Design review of the part built by this model. Coordinates are the model's own, in mm. A direction names the side the tool comes from. Coordinates: 2 decimals unless noted, no trailing zeros. Order: outer loops, then holes, each group sorted by start corner. A loop starts at its lowest first (then second) coordinate and runs counter-clockwise, first axis right, second up. Notation, with made-up numbers: (51, 33) - (81, 33) arc R19 ccw to (81, 47) - close; hole circle Ø6 at (14.5, 21). An arc over 180 degrees is marked (long way). Write each question's results on one line, items separated by ' | '. Start each with the question number.
```python
from build123d import *

# Parameters (mm, degrees)
F0_W        = 100
F0_H        = 260
F1_DEPTH    = 30
F3_R        = 5
F2_R        = 45
F4_DEPTH    = 20
F5_T        = 5
F5_T4_ANGLE = 180.000000001
F5_T6_ANGLE = 180.000000001


# Not quite as in the source:
# - a shell that OpenCascade refuses in one call is made with other operations: the cavity is built on its own and cut out


with BuildPart() as f1:
    # F0 (on Front) → F1 (new body)
    with BuildSketch(Plane.XZ):
        with Locations((-0.186801888, -30)):
            Rectangle(F0_W, F0_H)
    extrude(amount=-F1_DEPTH)

    # F3
    f3_edges = [f1.edges().sort_by_distance(p)[0] for p in [
        (49.813198, 0, -30),
        (-50.186802, 0, -30),
        (-0.186802, 30, 100),
    ]]
    fillet(f3_edges, radius=F3_R)

    # F2 (on Front) → F4 (join)
    with BuildSketch(Plane.XZ):
        with Locations((-0.186801888, 50)):
            Circle(F2_R)
    extrude(amount=F4_DEPTH)

    # F5: shell of thickness 5, made by hand


with BuildPart() as f5_core1:
    # F5_t2: copy of F1
    add(f1.part)

    # the walls: a layer under each face that stays
    f5_faces = [f5_core1.faces().sort_by_distance(p)[0] for p in [
        (-0.186801888, 12.5, 100),
        (49.813198112, 17.5, -30),
        (-30.186801888, 0, 91.6666666667),
        (-50.186801888, 17.5, -30),
        (-0.186801888, 30, -32.5),
        (-0.186801888, 0, -55),
        (-45.186801888, -10, 50),
        (-0.186801888, -20, 50),
    ]]
    thicken(f5_faces, amount=-F5_T, mode=Mode.SUBTRACT)

    # F5_s3 → F5_t4 (revolve, cut)
    with BuildSketch(Plane.XY.offset(50)):
        Polygon((44.863198112, -0.05), (44.813198112, 5), (39.813198112, 5), (39.813198112, 0), align=None)
    revolve(axis=Axis((-0.186801888, 0, 50), (0, -1, 0)), revolution_arc=F5_T4_ANGLE, mode=Mode.SUBTRACT)

    # F5_s5 → F5_t6 (revolve, cut)
    with BuildSketch(Plane.XY.offset(50)):
        Polygon((-45.236801888, -0.05), (-45.186801888, 5), (-40.186801888, 5), (-40.186801888, 0), align=None)
    revolve(axis=Axis((-0.186801888, 0, 50), (0, -1, 0)), revolution_arc=F5_T6_ANGLE, mode=Mode.SUBTRACT)


with BuildPart() as f1_1:
    add(f1.part)

    # what is left inside the walls is the cavity
    f5_cavity = [f5_core1.part.solids().sort_by_distance(p)[0] for p in [
        (-0.186802, 24.95, -75),
    ]]
    add(f5_cavity, mode=Mode.SUBTRACT)


solid = f1_1.part
```
(1) Clearance check with flat-ended pins moving along their axes: pin 1 (10 mm diameter, centred on x = 8.5, y = 19.5, fed in from -Z); pin 2 (5 mm diameter, centred on x = 24, y = -12, fed in from +Z); pin 3 (3 mm diameter, centred on x = -10.5, z = -130, fed in from -Y). State where each tip first meets the part, or that it passes through.
(2) Take a section at D-D (x = 9). State the section outline as (y, z) points, plus the area to 3 significant figures.
(3) Take a section at B-B (y = 20). State the section outline as (x, z) points.
(4) Take a section at C-C (x = 24). State the section outline as (y, z) points, plus the area to 3 significant figures.
(5) Mouldability with a two-part tool opening along X and no side actions: class faces 6 (the face through (-1, 15, 95)), 7 (the face through (48.387, 1.504, -28.18)), 8 (the face through (-48.76, 1.5, -28.18)), 9 (the face through (-1, 12, 100)) as +X half, -X half, draft (parallel to the pull), parting line (faces both ways), or undercut.
(6) Take a section at A-A (z = -25.5). State the section outline as (x, y) points, plus the area to 3 significant figures.
(7) Tool access review of faces 1 (the face through (-9.94, -9.86, 6.07)), 2 (the face through (-0.4, 0, 95.5)), 3 (the face through (-1, 30, -31)), 4 (the face through (-1, -15, 51)), 5 (the face through (-1, 5, -59)): name each direction out of +Z, -Z, +X, -X, +Y, -Y from which nothing blocks a thin tool from reaching the whole face with its end or side.
(8) To check wall thickness, follow line 1 along Y through (x, z) = (28, -13); line 2 along Y through (x, z) = (-23, 50); line 3 along X through (y, z) = (22, 55). State the ranges of each line that lie inside material, in increasing order. Write a range as [from, to].
Worked out:
1) pin 1: z = 95 | pin 2: z = 89.43 | pin 3: y = 0
2) outline: (-20, 5.95) - (0, 5.95) - (0, -160) - (5, -160) - (5, 11.07) - (-15, 11.07) - (-15, 88.93) - (5, 88.93) - (5, 95) - (25, 95) - (25, -160) - (30, -160) - (30, 95) arc R5 ccw to (25, 100) - (0, 100) - (0, 94.05) - (-20, 94.05) - close | area: 2,900 mm^2
3) outline: (-50.19, -160) - (-45.19, -160) - (-45.19, 95) - (44.81, 95) - (44.81, -160) - (49.81, -160) - (49.81, 100) - (-50.19, 100) - close
4) outline: (-20, 12.05) - (0, 12.05) - (0, -160) - (5, -160) - (5, 18.14) - (-15, 18.14) - (-15, 81.86) - (5, 81.86) - (5, 95) - (25, 95) - (25, -160) - (30, -160) - (30, 95) arc R5 ccw to (25, 100) - (0, 100) - (0, 87.95) - (-20, 87.95) - close | area: 2,940 mm^2
5) face 6: undercut | face 7: +X half | face 8: -X half | face 9: draft
6) outline: (-50.19, 5) arc R5 ccw to (-45.19, 0) - (44.81, 0) arc R5 ccw to (49.81, 5) - (49.81, 30) - (-50.19, 30) - close; hole (-45.19, 5) - (44.81, 5) - (44.81, 25) - (-45.19, 25) - close | area: 1,190 mm^2
7) face 1: -Y | face 2: +Z, -Y | face 3: +Z, -Z, +X, -X, +Y | face 4: none | face 5: -Z
8) line 1: [0, 5], [25, 30] | line 2: [-20, -15], [25, 30] | line 3: [-50.19, -45.19], [44.81, 49.81]
